Geometry check sheet. Reference: drawing and pictorial views, mm from the part's lowest x, y, z. Coordinates: 2 decimals unless noted, no trailing zeros. Write each loop counter-clockwise with the first axis right and the second up, starting at its lowest first coordinate (ties: lowest second). Pieces come first, ordered by that corner, then holes. Notation, with made-up numbers: (85, 42.25) - (130, 42.25) arc R14 cw to (130, 64.25) - close; hole circle Ø9 at (14.25, 14). An arc over 180 degrees is marked (long way). Use one line per item in the form item = value. Start each with the question number.
(1) Material ranges on line 1 (Y direction, x = 2.5, z = 1.75); line 2 (Y direction, x = 3.2, z = 3.8); line 3 (X direction, y = 2.7, z = 2.5), recorded low to high. Write a range as [from, to].
(2) Sectioned sample at B-B (z = 4.45). Record the cut outline in (x, y), and give its area (3 significant figures).
(3) Mould release check, pull along Y, two halves, no side actions. Record for the marked faces 1, 2, 3 and 4: released by +Y, released by -Y, zero draft, split by the parting line, or undercut.
(4) Sectioned sample at A-A (y = 2.5). Record the cut outline in (x, z).
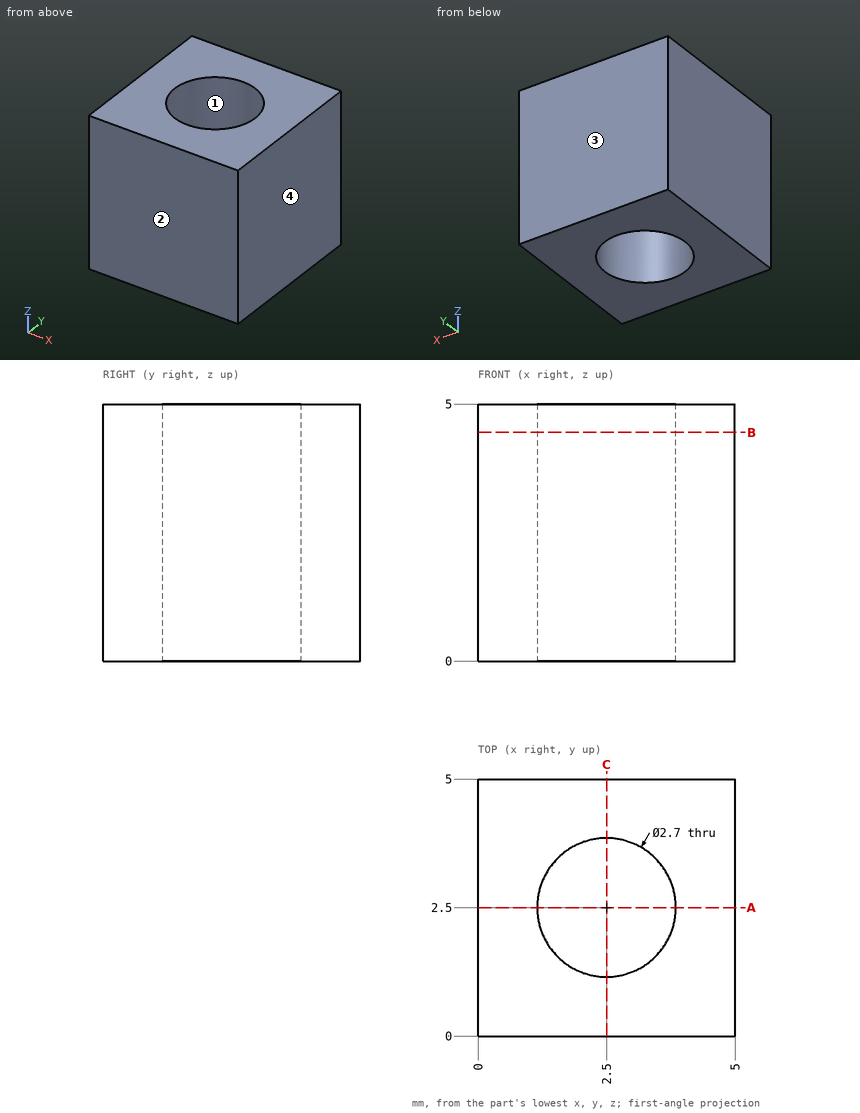
Answers below:
q1.line_1 = [0, 1.15], [3.85, 5]
q1.line_2 = [0, 1.35], [3.65, 5]
q1.line_3 = [0, 1.16], [3.84, 5]
q2.outline = (0, 0) - (5, 0) - (5, 5) - (0, 5) - close; hole circle Ø2.7 at (2.5, 2.5)
q2.area = 19.3 mm2
q3.face_1 = undercut
q3.face_2 = released by -Y
q3.face_3 = released by +Y
q3.face_4 = zero draft
q4.outline = (0, 0) - (1.15, 0) - (1.15, 5) - (0, 5) - close; (3.85, 0) - (5, 0) - (5, 5) - (3.85, 5) - close
